from build123d import *

# Parameters (mm, degrees)
SKETCH1_R                     = 177
SKETCH1_R_2                   = 2.2479
BOSS_EXTRUDE1_DEPTH           = 4.7625
SKETCH2_R                     = 1.7
JETSONHOLES_DEPTH             = 251.361102023
SKETCH3_R                     = 9.525
UART_WIRE_HOLE_DEPTH          = 251.361102023
SKETCH6_R                     = 1.7
SKETCH6_R_2                   = 8.89
NIMH_HOLES_DEPTH              = 251.361102023
SKETCH7_R                     = 1.7
IMU_HOLES_DEPTH               = 251.361102023
SKETCH8_R                     = 1.7
LEVEL2_3_STANDOFF_HOLES_DEPTH = 251.361102023
SKETCH9_R                     = 2.667
ZIP_TIES_DEPTH                = 251.361102023


with BuildPart() as part:
    # Sketch1 → Boss-Extrude1 (new body)
    with BuildSketch(Plane(origin=(0, 0, 0), x_dir=(1, 0, 0), z_dir=(0, 1, 0))):
        with Locations(Location((0, 0, 0), (0, 0, 90))):
            Circle(SKETCH1_R)
        with Locations(Location((-101.6, -101.6, 0), (0, 0, 90))):
            Circle(SKETCH1_R_2, mode=Mode.SUBTRACT)
        with Locations(Location((-101.6, 101.6, 0), (0, 0, 90))):
            Circle(SKETCH1_R_2, mode=Mode.SUBTRACT)
        with Locations(Location((101.6, 101.6, 0), (0, 0, 90))):
            Circle(SKETCH1_R_2, mode=Mode.SUBTRACT)
        with Locations(Location((101.6, -101.6, 0), (0, 0, 90))):
            Circle(SKETCH1_R_2, mode=Mode.SUBTRACT)
    extrude(amount=BOSS_EXTRUDE1_DEPTH)

    # Sketch2 → JetsonHoles (cut, through all)
    with BuildSketch(Plane(origin=(0, 4.7625, 0), x_dir=(1, 0, 0), z_dir=(0, 1, 0))):
        with Locations(Location((-53.213, 51.435, 0), (0, 0, 270))):
            Circle(SKETCH2_R)
        with Locations(Location((53.213, 51.435, 0), (0, 0, 270))):
            Circle(SKETCH2_R)
        with Locations(Location((-53.213, -51.435, 0), (0, 0, 270))):
            Circle(SKETCH2_R)
        with Locations(Location((53.213, -51.435, 0), (0, 0, 270))):
            Circle(SKETCH2_R)
    extrude(amount=-JETSONHOLES_DEPTH, mode=Mode.SUBTRACT)

    # Sketch3 → UART-Wire-Hole (cut, through all)
    with BuildSketch(Plane(origin=(0, 4.7625, 0), x_dir=(1, 0, 0), z_dir=(0, 1, 0))):
        with Locations(Location((-63.5, 12.7, 0), (0, 0, 270))):
            Circle(SKETCH3_R)
    extrude(amount=-UART_WIRE_HOLE_DEPTH, mode=Mode.SUBTRACT)

    # Sketch6 → NiMH_Holes (cut, through all)
    with BuildSketch(Plane(origin=(0, 4.7625, 0), x_dir=(1, 0, 0), z_dir=(0, 1, 0))):
        with Locations(Location((101.6, 60.96, 0), (0, 0, 270))):
            Circle(SKETCH6_R)
        with Locations(Location((76.2, -60.96, 0), (0, 0, 270))):
            Circle(SKETCH6_R)
        with Locations(Location((-101.6, -60.96, 0), (0, 0, 270))):
            Circle(SKETCH6_R)
        with Locations(Location((-76.2, 60.96, 0), (0, 0, 270))):
            Circle(SKETCH6_R)
        with Locations(Location((-50.8, 101.6, 0), (0, 0, 270))):
            Circle(SKETCH6_R_2)
        with Locations(Location((50.8, 101.6, 0), (0, 0, 270))):
            Circle(SKETCH6_R_2)
    extrude(amount=-NIMH_HOLES_DEPTH, mode=Mode.SUBTRACT)

    # Sketch7 → IMU_Holes (cut, through all)
    with BuildSketch(Plane(origin=(0, 4.7625, 0), x_dir=(1, 0, 0), z_dir=(0, 1, 0))):
        with Locations(Location((-9.55000005, 8.162499942, 0), (0, 0, 270))):
            Circle(SKETCH7_R)
        with Locations(Location((9.54999995, 8.162499942, 0), (0, 0, 270))):
            Circle(SKETCH7_R)
        with Locations(Location((-9.55000005, -8.162500058, 0), (0, 0, 270))):
            Circle(SKETCH7_R)
        with Locations(Location((9.54999995, -8.162500058, 0), (0, 0, 270))):
            Circle(SKETCH7_R)
    extrude(amount=-IMU_HOLES_DEPTH, mode=Mode.SUBTRACT)

    # Sketch8 → Level2_3_Standoff_holes (cut, through all)
    with BuildSketch(Plane(origin=(0, 4.7625, 0), x_dir=(1, 0, 0), z_dir=(0, 1, 0))):
        with Locations(Location((-114.3, -82.55, 0), (0, 0, 270))):
            Circle(SKETCH8_R)
        with Locations(Location((-114.3, 82.55, 0), (0, 0, 270))):
            Circle(SKETCH8_R)
        with Locations(Location((114.3, 82.55, 0), (0, 0, 270))):
            Circle(SKETCH8_R)
        with Locations(Location((114.3, -82.55, 0), (0, 0, 270))):
            Circle(SKETCH8_R)
    extrude(amount=-LEVEL2_3_STANDOFF_HOLES_DEPTH, mode=Mode.SUBTRACT)

    # Sketch9 → Zip Ties (cut, through all)
    with BuildSketch(Plane(origin=(0, 4.7625, 0), x_dir=(1, 0, 0), z_dir=(0, 1, 0))):
        with Locations(Location((0, -141.44, 0), (0, 0, 270))):
            Circle(SKETCH9_R)
        with Locations(Location((-83.136346084, -114.427363684, 0), (0, 0, 270))):
            Circle(SKETCH9_R)
        with Locations(Location((-134.517433665, -43.707363684, 0), (0, 0, 270))):
            Circle(SKETCH9_R)
        with Locations(Location((-134.517433665, 43.707363684, 0), (0, 0, 270))):
            Circle(SKETCH9_R)
        with Locations(Location((-83.136346084, 114.427363684, 0), (0, 0, 270))):
            Circle(SKETCH9_R)
        with Locations(Location((0, 141.44, 0), (0, 0, 270))):
            Circle(SKETCH9_R)
        with Locations(Location((83.136346084, 114.427363684, 0), (0, 0, 270))):
            Circle(SKETCH9_R)
        with Locations(Location((134.517433665, 43.707363684, 0), (0, 0, 270))):
            Circle(SKETCH9_R)
        with Locations(Location((134.517433665, -43.707363684, 0), (0, 0, 270))):
            Circle(SKETCH9_R)
        with Locations(Location((83.136346084, -114.427363684, 0), (0, 0, 270))):
            Circle(SKETCH9_R)
    extrude(amount=-ZIP_TIES_DEPTH, mode=Mode.SUBTRACT)


solid = part.part
Geometry check sheet. Reference: the model listing, model coordinates, mm. Give positions to 0.01 mm unless a question says otherwise; leave off trailing zeros. Order: outer loops, then holes, each group sorted by start corner. A loop starts at its lowest first (then second) coordinate and runs counter-clockwise, first axis right, second up. Notation, with made-up numbers: M 56,34 L 82,34 A22 cw 82,58 Z; hole C -33,-18 d2. An arc over 180 degrees is marked long. Use a Markdown table: item, result.
Item 1: Depth check by flat-ended pin: P1, Ø20.5, axis at x = -50.8, z = -101.6, coming from the +Y side. Enter the tip coordinate at first touch or a pass-through.
Answers follow:
| item | result |
|---|---|
| P1 | stops at y = 4.76 |
Item 2: Material ranges on line 1 along X through (y, z) = (3.85, -109); line 2 along Z through (x, y) = (-101.6, 1.05); line 3 along Z through (x, y) = (-9.55, 3.6), recorded low to high.
Answers follow:
| item | result |
|---|---|
| line 1 | x = -139.46 to -55.73, -45.87 to 45.87, 55.73 to 139.46 |
| line 2 | z = -144.94 to -103.85, -99.35 to 59.26, 62.66 to 99.35, 103.85 to 144.94 |
| line 3 | z = -176.74 to -9.86, -6.46 to 6.46, 9.86 to 176.74 |
Item 3: Section check C-C (x = -37). Record the cut outline in (y, z).
Answers follow:
| item | result |
|---|---|
| outline | M 0,-173.09 L 4.76,-173.09 L 4.76,173.09 L 0,173.09 Z |
Item 4: Section check B-B (z = -149). Record the cut outline in (x, y), and give its area (3 significant figures).
Answers follow:
| item | result |
|---|---|
| outline | M -95.54,0 L 95.54,0 L 95.54,4.76 L -95.54,4.76 Z |
| area | 910 mm2 |
Item 5: Section check A-A (y = 1.7). State how many separate pieces and enclosed holes the cut face has, and give its area (3 significant figures).
Answers follow:
| item | result |
|---|---|
| separate pieces | 1 |
| enclosed holes | 33 |
| area | 97,200 mm2 |
Item 6: Draft check along X on faces 1 (the cylindrical face through (51.19, 2.41, -110.48)), 2 (the flat face through (-2, 4.762, 2)), 3 (the cylindrical face through (172.79, 2.35, 38.37)). Enter one of: +X half, -X half, draft (parallel to the pull), parting line (faces both ways), or undercut.
Answers follow:
| item | result |
|---|---|
| face 1 | undercut |
| face 2 | draft |
| face 3 | parting line |
